Job drawing, mm, ordinate dimensions from the low corner. One solid piece. A direction names the side the tool comes from. Coordinates: 2 decimals unless noted, no trailing zeros. Loops run counter-clockwise (first coordinate to the right, second up) from the corner with the lowest first, then second, coordinate; pieces in that order, holes last. Notation, with made-up numbers: (68.5, 0.25) - (83.5, 0.25) arc R11 cw to (83.5, 15.25) - close; hole circle Ø8 at (-20.5, 86). An arc over 180 degrees is marked (long way). Use a Markdown table: item, result. Add a question column.
1) Drop flat-ended pins along their axis: P1, Ø5.5, axis at x = 55.4, z = 30, coming from the +Y side; P2, Ø5, axis at x = 32, z = 27.5, coming from the +Y side. Give the stop position or say it passes through.
2) Tool access for the marked faces 1 and 2: list every direction of +Z, -Z, +X, -X, +Y, -Y with a clear straight run to the whole face (end or side of a thin tool).
3) Band-saw the part on D-D (z = 40.5). Give the cut face in (x, y).
4) Pull direction Z, two halves, no side cores. Call the marked faces 3, 4 and 5: +Z half, -Z half, draft (parallel to the pull), parting line (faces both ways), or undercut.
5) Band-saw the part on B-B (x = 55.4). Give the cut face in (y, z), plus the area to 3 significant figures.
6) Band-saw the part on A-A (z = 30). Give the cut face in (x, y).
7) Band-saw the part on C-C (y = 5). Give the cut face in (x, z).
8) Probe probe 1 along Z at (x, y) = (55.4, 3.75); probe 2 along X at (y, z) = (3.25, 30); probe 3 along Z at (x, y) = (52.5, 3). List the from-to ranges inside material, lowest first. Write a range as [from, to].
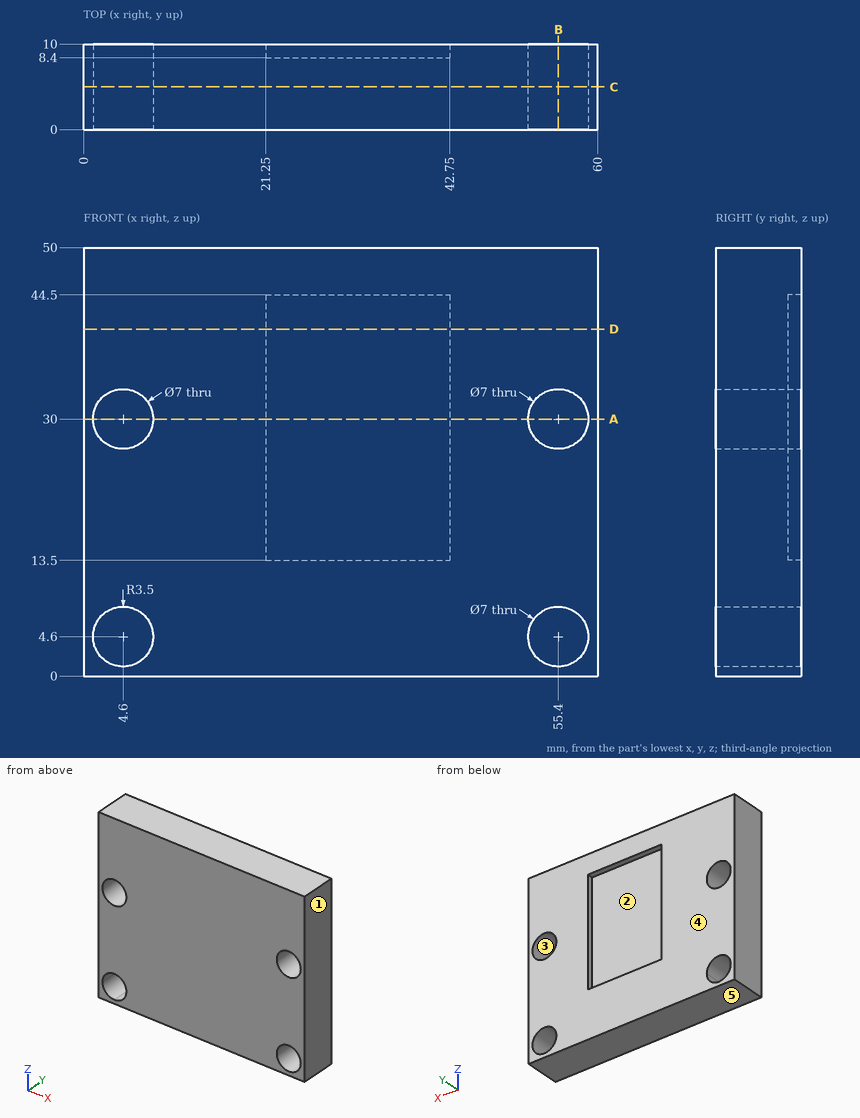
Answer block:
| question | item | result |
|---|---|---|
| 1 | P1 | through |
| 1 | P2 | y = 8.4 |
| 2 | face 1 | +Z, -Z, +X, +Y, -Y |
| 2 | face 2 | +Y |
| 3 | outline | (0, 0) - (60, 0) - (60, 10) - (42.75, 10) - (42.75, 8.4) - (21.25, 8.4) - (21.25, 10) - (0, 10) - close |
| 4 | face 3 | undercut |
| 4 | face 4 | draft |
| 4 | face 5 | -Z half |
| 5 | outline | (0, 0) - (10, 0) - (10, 1.1) - (0, 1.1) - close; (0, 8.1) - (10, 8.1) - (10, 26.5) - (0, 26.5) - close; (0, 33.5) - (10, 33.5) - (10, 50) - (0, 50) - close |
| 5 | area | 360 mm2 |
| 6 | outline | (0, 0) - (1.1, 0) - (1.1, 10) - (0, 10) - close; (8.1, 0) - (51.9, 0) - (51.9, 10) - (42.75, 10) - (42.75, 8.4) - (21.25, 8.4) - (21.25, 10) - (8.1, 10) - close; (58.9, 0) - (60, 0) - (60, 10) - (58.9, 10) - close |
| 7 | outline | (0, 0) - (60, 0) - (60, 50) - (0, 50) - close; hole circle Ø7 at (4.6, 4.6); hole circle Ø7 at (4.6, 30); hole circle Ø7 at (55.4, 4.6); hole circle Ø7 at (55.4, 30) |
| 8 | probe 1 | [0, 1.1], [8.1, 26.5], [33.5, 50] |
| 8 | probe 2 | [0, 1.1], [8.1, 51.9], [58.9, 60] |
| 8 | probe 3 | [0, 2.64], [6.56, 28.04], [31.96, 50] |
